For this review, take the finished solid that the model builds, in its own axes (mm). Face numbers are marked on the shaded views. A direction names the side the tool comes from. Give positions to 0.01 mm unless a question says otherwise; leave off trailing zeros. Write each loop counter-clockwise with the first axis right and the second up, starting at its lowest first coordinate (ties: lowest second). Pieces come first, ordered by that corner, then holes. Notation, with made-up numbers: M 86,3 L 132,3 A16 ccw 132,13 Z; hole C 55,3.5 d9. An arc over 180 degrees is marked long. Write item = value, one per line.
```python
from build123d import *

# Parameters (mm, degrees)
SKETCH1_W           = 12
SKETCH1_H           = 12
BOSS_EXTRUDE1_DEPTH = 3.3
SKETCH2_R           = 3.25
BOSS_EXTRUDE2_DEPTH = 1.6
BOSS_EXTRUDE2_TAPER = 6


with BuildPart() as part:
    # Sketch1 → Boss-Extrude1 (new body)
    with BuildSketch(Plane(origin=(0, 0, 0), x_dir=(1, 0, 0), z_dir=(0, 1, 0))):
        Rectangle(SKETCH1_W, SKETCH1_H)
    extrude(amount=BOSS_EXTRUDE1_DEPTH)

    # Sketch2 → Boss-Extrude2 (add)
    with BuildSketch(Plane(origin=(0, 3.3, 0), x_dir=(1, 0, 0), z_dir=(0, 1, 0))):
        Circle(SKETCH2_R)
    extrude(amount=BOSS_EXTRUDE2_DEPTH, taper=BOSS_EXTRUDE2_TAPER)


solid = part.part
```
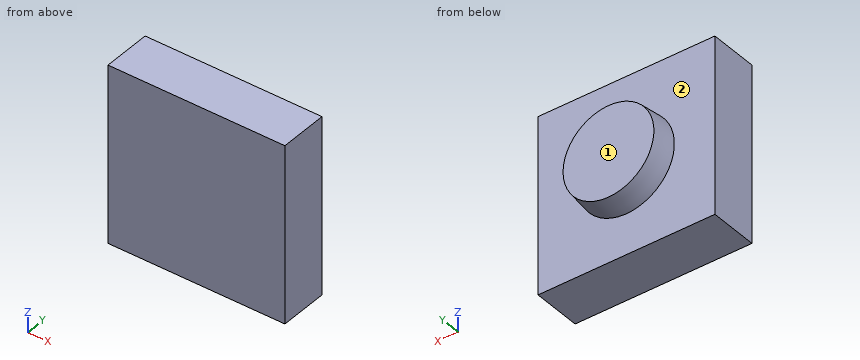
1. We need section C-C, the plane y = 3.8. Write out the cut boundary in (x, z), then the cut area to 3 significant figures.
Responses:
outline = C 0,0 d6.39
area = 32.1 mm2
2. We need section B-B, the plane z = 4. Write out the cut boundary in (x, y), then the cut area to 3 significant figures.
Responses:
outline = M -6,0 L 6,0 L 6,3.3 L -6,3.3 Z
area = 39.6 mm2
3. For line 1 along Y through (x, z) = (5.75, -2); line 2 along Z through (x, y) = (-0.5, 4.3); line 3 along Z through (x, y) = (2, 3.35), list the stretches that pass through material, from the lowest coordinate up. Write a range as from..to.
Responses:
line_1 = 0..3.3
line_2 = -3.1..3.1
line_3 = -2.56..2.56
4. We need section A-A, the plane x = 0. Write out the cut boundary in (y, z).
Responses:
outline = M 0,-6 L 3.3,-6 L 3.3,-3.25 L 4.9,-3.08 L 4.9,3.08 L 3.3,3.25 L 3.3,6 L 0,6 Z
5. Machinability: for the marked faces 1 and 2, which of the approach directions +Z, -Z, +X, -X, +Y, -Y give a long, thin tool a straight path to every point of the face, cutting with its end or side? Answer none if there is none.
Responses:
face_1 = +Z, -Z, +X, -X, +Y
face_2 = +Y
